Design review of the part built by this model. Coordinates are the model's own, in mm. Face numbers are marked on the shaded views. A direction names the side the tool comes from. Give positions to 0.01 mm unless a question says otherwise; leave off trailing zeros. Write each loop counter-clockwise with the first axis right and the second up, starting at its lowest first coordinate (ties: lowest second). Pieces come first, ordered by that corner, then holes.
```python
from build123d import *

# Parameters (mm, degrees)
SKETCH_1_W          = 210
SKETCH_1_H          = 132
EXTRUDE_1_DEPTH     = 1
SKETCH_3_W          = 1
SKETCH_3_H          = 132
EXTRUDE_2_DEPTH     = 81
SKETCH_2_R          = 2
CUT_EXTRUDE_1_DEPTH = 1


with BuildPart() as part:
    # 草图1 → 凸台-拉伸1 (new body)
    with BuildSketch(Plane.XY):
        Rectangle(SKETCH_1_W, SKETCH_1_H)
    extrude(amount=EXTRUDE_1_DEPTH)

    # 草图3 → 凸台-拉伸2 (add)
    with BuildSketch(Plane.XY.offset(1)):
        with Locations((104.5, 0)):
            Rectangle(SKETCH_3_W, SKETCH_3_H)
    extrude(amount=EXTRUDE_2_DEPTH)

    # 草图2 → 切除-拉伸1 (cut)
    with BuildSketch(Plane.XY.offset(1)):
        with Locations((-75, 63)):
            Circle(SKETCH_2_R)
        with Locations((75, 63)):
            Circle(SKETCH_2_R)
    extrude(amount=-CUT_EXTRUDE_1_DEPTH, mode=Mode.SUBTRACT)


solid = part.part
```
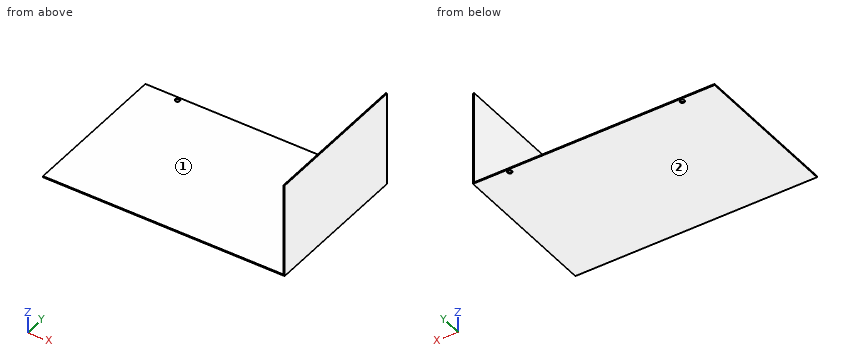
(1) Tool access review of the marked faces 1 and 2: name each direction out of +Z, -Z, +X, -X, +Y, -Y from which nothing blocks a thin tool from reaching the whole face with its end or side.
Resolved:
face 1: +Z, -X, +Y, -Y
face 2: -Z, +X, -X, +Y, -Y
(2) Consider section C-C, the plane z = 67.5. Give the boundary of the cut face in (x, y), then the cut area to 3 significant figures.
Resolved:
outline: (104, -66) - (105, -66) - (105, 66) - (104, 66) - close
area: 132 mm2
(3) To check wall thickness, follow L1, parallel to Y at x = 75, z = 0.75; L2, parallel to X at y = -46.5, z = 27.5; L3, parallel to Z at x = 16, y = 30. State the ranges of each line that lie inside material, in increasing order.
Resolved:
L1: y = -66 to 61, 65 to 66
L2: x = 104 to 105
L3: z = 0 to 1
(4) Clearance check with flat-ended pins moving along their axes: P1, Ø10, axis at x = -78, y = -49, coming from the -Z side; P2, Ø1.5, axis at x = 6, y = -14.5, coming from the +Z side; P3, Ø1, axis at y = 46.5, z = 61.5, coming from the -X side. State where each tip first meets the part, or that it passes through.
Resolved:
P1: stops at z = 0
P2: stops at z = 1
P3: stops at x = 104
(5) Consider section B-B, the plane x = -46. Give the boundary of the cut face in (y, z).
Resolved:
outline: (-66, 0) - (66, 0) - (66, 1) - (-66, 1) - close
(6) Consider section A-A, the plane y = 23. Give the boundary of the cut face in (x, z), then the cut area to 3 significant figures.
Resolved:
outline: (-105, 0) - (105, 0) - (105, 82) - (104, 82) - (104, 1) - (-105, 1) - close
area: 291 mm2
